For this review, take the finished solid that the model builds, in its own axes (mm). Round coordinates to 2 decimals unless told otherwise and drop trailing zeros. Loops run counter-clockwise (first coordinate to the right, second up) from the corner with the lowest first, then second, coordinate; pieces in that order, holes last.
1) Take a section at B-B (x = 71.5). State the section outline as (y, z) points (3 decimals).
2) Take a section at D-D (y = -19). State the section outline as (x, z) points (3 decimals), then the cut area to 3 significant figures.
3) Take a section at A-A (y = 0). State the section outline as (x, z) points (3 decimals).
4) Take a section at C-C (z = 0.75). State the section outline as (x, y) points (3 decimals).
5) Wall thickness on L1, parallel to Y at x = 0, z = 1.8; L2, parallel to X at y = 7.5, z = 2.1; L3, parallel to X at y = 33.5, z = 0.8: over which ranges is each line inside the solid? List them lowest first.
6) Insertion check: pin 1 (1 mm diameter, centred on x = -4, z = 1, fed in from +Y). The pin has a flat end and moves straight along its axis. Give the tip position at first contact, or say it passes through.
```python
from build123d import *

# Parameters (mm, degrees)
SKETCH1_R           = 83.4771
SKETCH1_R_2         = 3.175
BOSS_EXTRUDE1_DEPTH = 3.175


with BuildPart() as part:
    # Sketch1 → Boss-Extrude1 (new body)
    with BuildSketch(Plane.XY):
        with BuildLine():
            Line((-15.854735322, -44.594342032), (15.852600775, -44.594342032))
            ThreePointArc((15.852600775, -44.594342032), (49.382027762, -50.630069264), (78.701832464, -67.979464917))
            ThreePointArc((78.701832464, -67.979464917), (227.246053, 0), (78.701832464, 67.979464917))
            ThreePointArc((78.701832464, 67.979464917), (49.382027762, 50.630069264), (15.852600775, 44.594342032))
            Line((15.852600775, 44.594342032), (-15.854735322, 44.594342032))
            ThreePointArc((-15.854735322, 44.594342032), (-49.384162309, 50.630069264), (-78.703967011, 67.979464917))
            ThreePointArc((-78.703967011, 67.979464917), (-227.248187547, 0), (-78.703967011, -67.979464917))
            ThreePointArc((-78.703967011, -67.979464917), (-49.384162309, -50.630069264), (-15.854735322, -44.594342032))
        make_face()
        with Locations((137.418953, 0)):
            Circle(SKETCH1_R, mode=Mode.SUBTRACT)
        with Locations((-137.421087547, 0)):
            Circle(SKETCH1_R, mode=Mode.SUBTRACT)
        with Locations((0, 28.575000036)):
            Circle(SKETCH1_R_2, mode=Mode.SUBTRACT)
    extrude(amount=BOSS_EXTRUDE1_DEPTH)


solid = part.part
```
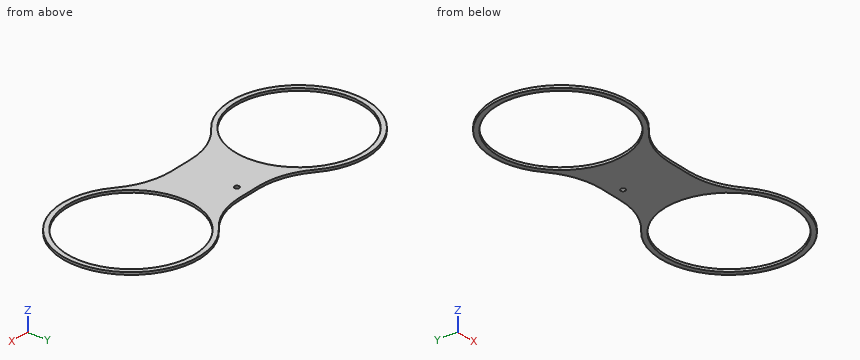
Response:
1. outline: (-62.334, 0) - (-51.216, 0) - (-51.216, 3.175) - (-62.334, 3.175) - close; (51.216, 0) - (62.334, 0) - (62.334, 3.175) - (51.216, 3.175) - close
2. outline: (-225.216, 0) - (-218.707, 0) - (-218.707, 3.175) - (-225.216, 3.175) - close; (-56.135, 0) - (56.133, 0) - (56.133, 3.175) - (-56.135, 3.175) - close; (218.705, 0) - (225.214, 0) - (225.214, 3.175) - (218.705, 3.175) - close
2. area: 398 mm2
3. outline: (-227.248, 0) - (-220.898, 0) - (-220.898, 3.175) - (-227.248, 3.175) - close; (-53.944, 0) - (53.942, 0) - (53.942, 3.175) - (-53.944, 3.175) - close; (220.896, 0) - (227.246, 0) - (227.246, 3.175) - (220.896, 3.175) - close
4. outline: (-78.704, -67.979) arc R96.149 cw to (-15.855, -44.594) - (15.853, -44.594) arc R96.149 cw to (78.702, -67.979) arc R89.827 ccw (long way) to (78.702, 67.979) arc R96.149 cw to (15.853, 44.594) - (-15.855, 44.594) arc R96.149 cw to (-78.704, 67.979) arc R89.827 ccw (long way) to start; hole circle Ø166.954 at (-137.421, 0); hole circle Ø6.35 at (0, 28.575); hole circle Ø166.954 at (137.419, 0)
5. L1: y = -44.59 to 25.4, 31.75 to 44.59
5. L2: x = -226.93 to -220.56, -54.28 to 54.28, 220.56 to 226.93
5. L3: x = -220.77 to -213.88, -60.96 to 60.96, 213.88 to 220.77
6. pin 1: stops at y = 44.59
